Verification items for this drawing (mm, ordinates from the low corner). Give positions to 0.01 mm unless a question says otherwise; leave off trailing zeros. Loops run counter-clockwise (first coordinate to the right, second up) from the corner with the lowest first, then second, coordinate; pieces in that order, holes last. Notation, with made-up numbers: (28.25, 74.25) -> (60.25, 74.25) arc R31 ccw to (60.25, 103.25) -> close; hole circle Ø10 at (-22, 53.5). An arc over 180 degrees is marked (long way). Answer as a JSON object with one key per item and string values.
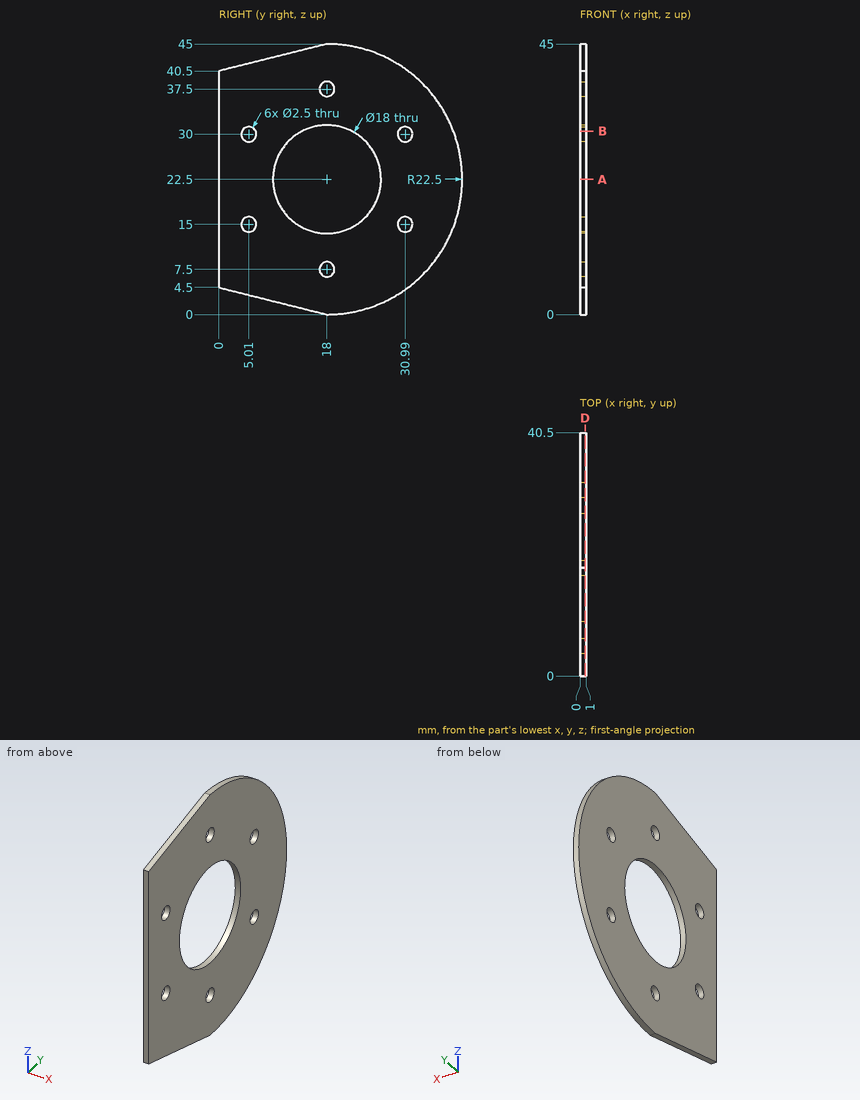
1) Section check A-A on z = 22.5. Record the cut outline in (x, y).
Geometry check:
{"outline": "(0, 0) -> (1, 0) -> (1, 9) -> (0, 9) -> close; (0, 27) -> (1, 27) -> (1, 40.5) -> (0, 40.5) -> close"}
2) Material ranges on line 1 along Y through (x, z) = (0.7, 22.5); line 2 along Y through (x, z) = (0.9, 15) (1 decimal); line 3 along Z through (x, y) = (0.1, 5), recorded low to high. Write a range as from..to.
Geometry check:
{"line 1": "y = 0..9, 27..40.5", "line 2": "y = 0..3.8, 6.3..13, 23..29.7, 32.2..39.2", "line 3": "z = 3.25..13.75, 16.25..28.75, 31.25..41.75"}
3) Depth check by flat-ended pin: P1, Ø4, axis at y = 5.01, z = 30, coming from the +X side; P2, Ø2, axis at y = 18, z = 7.5, coming from the +X side. Enter the tip coordinate at first touch or a pass-through.
Geometry check:
{"P1": "stops at x = 1", "P2": "passes through"}
4) Section check D-D on x = 0.8. Record the cut outline in (y, z).
Geometry check:
{"outline": "(0, 4.5) -> (18, 0) arc R22.5 ccw to (18, 45) -> (0, 40.5) -> close; hole circle Ø2.5 at (5.01, 15); hole circle Ø2.5 at (5.01, 30); hole circle Ø18 at (18, 22.5); hole circle Ø2.5 at (18, 7.5); hole circle Ø2.5 at (18, 37.5); hole circle Ø2.5 at (30.99, 15); hole circle Ø2.5 at (30.99, 30)"}
5) Section check B-B on z = 30.5. Record the cut outline in (x, y) (1 decimal), plus the area to 3 significant figures.
Geometry check:
{"outline": "(0, 0) -> (1, 0) -> (1, 3.9) -> (0, 3.9) -> close; (0, 6.2) -> (1, 6.2) -> (1, 13.9) -> (0, 13.9) -> close; (0, 22.1) -> (1, 22.1) -> (1, 29.8) -> (0, 29.8) -> close; (0, 32.1) -> (1, 32.1) -> (1, 39) -> (0, 39) -> close", "area": "26.2 mm2"}
